Input: part model. Units: mm. Frame: model coordinates. Face numbers are marked on the shaded views. A direction names the side the tool comes from. Coordinates: 2 decimals unless noted, no trailing zeros. Loops run counter-clockwise (first coordinate to the right, second up) from the corner with the lowest first, then second, coordinate; pieces in that order, holes last. Notation, with made-up numbers: (48, 61.25) - (76, 61.25) arc R20 cw to (76, 87.25) - close; hole circle Ø2 at (88.5, -37). An arc over 180 degrees is marked (long way). Use a Markdown table: item, result. Add a question column.
1. Section query C-C on x = 10.5. Return the cut outline in (y, z).
2. Access query for the marked faces 1 and 2. Directions: +Z, -Z, +X, -X, +Y, -Y. A direction counts if a zero-diameter tool reaches every point of the face in a straight line with its end or side. Return the directions, or none.
3. Ray query, L1, parallel to Y at x = 21, z = 2.25; L2, parallel to X at y = 16.5, z = -1.75; L3, parallel to X at y = 35, z = 5.75. Return the intervals inside material, ascending. Write a range as [from, to].
4. Section query D-D on z = -3.75. Return the cut outline in (x, y), then the cut area to 3 significant figures.
5. Contact query for flat-ended pins moving along their axis: P1, Ø1, axis at x = 10.5, y = -0.5, coming from the +Z side; P2, Ø12, axis at x = 6.5, y = -1.5, coming from the -Z side; P3, Ø13.5, axis at x = 27.5, z = 7, coming from the +Y side. Output: stop coordinate, or through.
6. Section query B-B on y = -2.5. Return the cut outline in (x, z).
7. Section query A-A on z = 3.75. Return the cut outline in (x, y).
```python
from build123d import *

# Parameters (mm, degrees)
F0_R     = 14.8676194835
F1_DEPTH = 63.81162256
F2_DEPTH = 53.6982640624
F4_DEPTH = 64.7173374891


with BuildPart() as f1:
    # F0 (on Front) → F1 (new body)
    with BuildSketch(Plane.XZ):
        with Locations((-0.3426838666, -0.586660404)):
            Circle(F0_R)
    extrude(amount=F1_DEPTH)

    # F2 (add): a face of the model
    f2_faces = [f1.faces().sort_by_distance(p)[0] for p in [
        (-0.3426838666, 0, -0.586660404),
    ]]
    extrude(f2_faces, amount=F2_DEPTH)

    # F3 (on face) → F4 (join)
    with BuildSketch(Plane.XZ.offset(63.81162256)):
        with BuildLine():
            ThreePointArc((7.2291272221, 12.2084084096), (12.4249878258, 7.0312572026), (14.5133566111, 0))
            Line((14.5133566111, 0), (45.0522339435, 0))
            Line((45.0522339435, 0), (7.2291272221, 12.2084084096))
        make_face()
    extrude(amount=-F4_DEPTH)


solid = f1.part
```
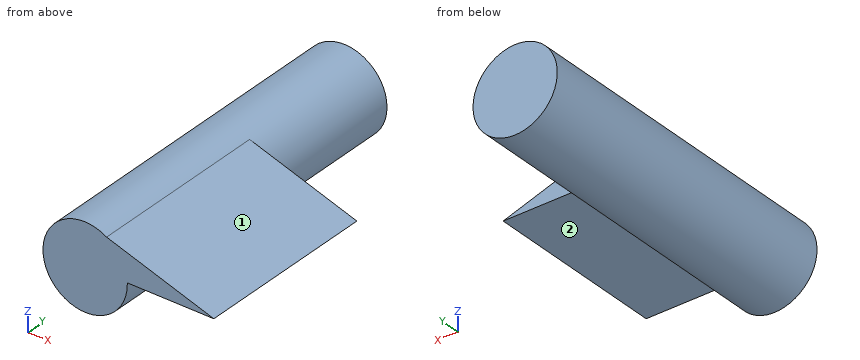
Resolved:
| question | item | result |
|---|---|---|
| 1 | outline | (-63.81, -10.76) - (53.7, -10.76) - (53.7, 9.59) - (0.91, 9.59) - (0.91, 11.15) - (-63.81, 11.15) - close |
| 2 | face 1 | +Z, +X, +Y, -Y |
| 2 | face 2 | -Z, +X, +Y, -Y |
| 3 | L1 | [-63.81, 0.91] |
| 3 | L2 | [-15.16, 14.48] |
| 3 | L3 | [-13.79, 13.11] |
| 4 | outline | (-14.87, -63.81) - (14.18, -63.81) - (14.18, 53.7) - (-14.87, 53.7) - close |
| 4 | area | 3,410 mm² |
| 5 | P1 | z = 11.31 |
| 5 | P2 | z = -15.43 |
| 5 | P3 | y = 0.91 |
| 6 | outline | (7.23, 12.21) arc R14.87 ccw (long way) to (14.51, 0) - (45.05, 0) - close |
| 7 | outline | (-14.56, -63.81) - (33.43, -63.81) - (33.43, 0.91) - (13.88, 0.91) - (13.88, 53.7) - (-14.56, 53.7) - close |
